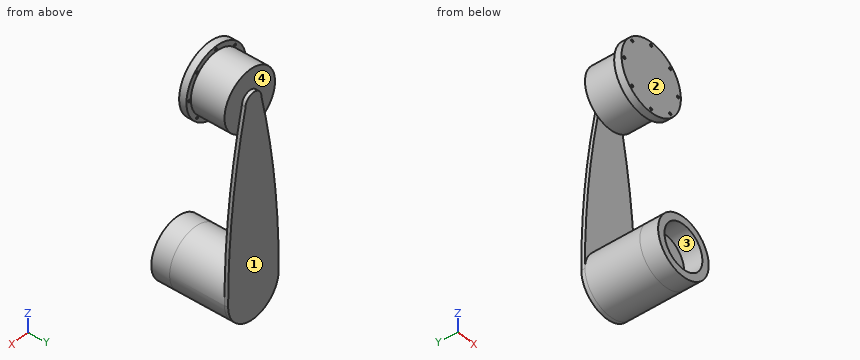
```python
from build123d import *
from build123d.topology import SkipClean

# Parameters (mm, degrees)
SKETCH_1_R          = 40
EXTRUDE_1_DEPTH     = 50
EXTRUDE_1_2_DEPTH   = 50
EXTRUDE_START       = 5
SKETCH_2_R          = 40
EXTRUDE_2_DEPTH     = 5
EXTRUDE_3_DEPTH     = 5
EXTRUDE_START_2     = -5
SKETCH_5_R          = 40
EXTRUDE_4_DEPTH     = 5
SKETCH_7_R          = 2
SKETCH_7_R_2        = 4
CUT_EXTRUDE_2_DEPTH = 10
CUT_EXTRUDE_START   = -59.05
SKETCH_9_R          = 40
CUT_EXTRUDE_4_DEPTH = 54.05
SKETCH_10_R         = 47
EXTRUDE_5_DEPTH     = 10
CUT_EXTRUDE_5_REACH = 302.04
SKETCH_11_R         = 1.75
CUT_EXTRUDE_START_2 = -80
SKETCH_12_R         = 39.999999969
CUT_EXTRUDE_6_DEPTH = 20
SKETCH_14_R         = 40
EXTRUDE_6_DEPTH     = 5
CUT_EXTRUDE_8_DEPTH = 10
CUT_EXTRUDE_9_DEPTH = 5
EXTRUDE_8_DEPTH     = 5
SKETCH_13_R         = 39.999999969
SKETCH_13_R_2       = 29.999999969
EXTRUDE_1_3_DEPTH   = 25


with BuildPart() as part:
    # Sketch 1 → Extrude 1 (new, symmetric)
    with BuildSketch(Plane(origin=(0, 0, 0), x_dir=(1, 0, 0), z_dir=(0, 1, 0))):
        with Locations(Location((0, 0, 0), (0, 0, 270))):
            Circle(SKETCH_1_R)
    extrude(amount=EXTRUDE_1_DEPTH, both=True)



with BuildPart() as body_2:
    # Sketch 1 → Extrude 1 2 (new, symmetric)
    with BuildSketch(Plane(origin=(0, 0, 0), x_dir=(1, 0, 0), z_dir=(0, 1, 0))):
        with Locations(Location((0, 250, 0), (0, 0, 270))):
            Circle(SKETCH_1_R)
    extrude(amount=EXTRUDE_1_2_DEPTH, both=True)


with BuildPart() as part_1:
    add(part.part)

    add(body_2.part)  # Extrude 2 merges body 2
    # Sketch 2 → Extrude 2 (add)
    with BuildSketch(Plane(origin=(0, 50, 0), x_dir=(1, 0, 0), z_dir=(0, 1, 0)).offset(EXTRUDE_START)):
        with BuildLine():
            ThreePointArc((39.999999755, 249.995569239), (-0.00221538, 210.000000061), (-40, 250))
            Line((-40, 250), (-40, 0))
            ThreePointArc((-40, 0), (-0.527343072, -39.996523715), (39.986095464, -1.054594484))
            Line((39.986095464, -1.054594484), (39.999999755, 249.995569239))
        make_face()
        with Locations(Location((0, 250, 0), (0, 0, 180))):
            Circle(SKETCH_2_R)
    extrude(amount=-EXTRUDE_2_DEPTH)

    # Sketch 3 → Extrude 3 (add)
    with BuildSketch(Plane(origin=(0, -50, 0), x_dir=(-1, 0, 0), z_dir=(0, -1, 0))):
        with BuildLine():
            Line((40, 0), (40, 250))
            ThreePointArc((40, 250), (0, 290), (-40, 250))
            Line((-40, 250), (-40, 0))
            ThreePointArc((-40, 0), (0, -40), (40, 0))
        make_face()
    extrude(amount=EXTRUDE_3_DEPTH)

    # Sketch 5 → Extrude 4 (add)
    with BuildSketch(Plane.XZ.offset(55).offset(EXTRUDE_START_2)):
        with Locations(Location((0, 0, 0), (0, 0, 180))):
            Circle(SKETCH_5_R)
    extrude(amount=EXTRUDE_4_DEPTH)

    # Sketch 7 → Cut-Extrude 2 (cut)
    with BuildSketch(Plane.XZ.offset(55)):
        with Locations(Location((17.25, -250, 0), (0, 0, 270))):
            Circle(SKETCH_7_R)
        with Locations(Location((8.625, -264.938938215, 0), (0, 0, 270))):
            Circle(SKETCH_7_R)
        with Locations(Location((-8.625, -264.938938215, 0), (0, 0, 270))):
            Circle(SKETCH_7_R)
        with Locations(Location((-17.25, -250, 0), (0, 0, 270))):
            Circle(SKETCH_7_R)
        with Locations(Location((-8.625, -235.061061785, 0), (0, 0, 270))):
            Circle(SKETCH_7_R)
        with Locations(Location((8.625, -235.061061785, 0), (0, 0, 270))):
            Circle(SKETCH_7_R)
        with Locations(Location((0, -250, 0), (0, 0, 270))):
            Circle(SKETCH_7_R_2)
    extrude(amount=-CUT_EXTRUDE_2_DEPTH, mode=Mode.SUBTRACT)

    # Sketch 9 → Cut-Extrude 4 (cut)
    with BuildSketch(Plane.XZ.offset(55).offset(CUT_EXTRUDE_START)):
        with Locations(Location((0, 0, 0), (0, 0, 270))):
            Circle(SKETCH_9_R)
    extrude(amount=CUT_EXTRUDE_4_DEPTH, mode=Mode.SUBTRACT)

    # Sketch 10 → Extrude 5 (add)
    with BuildSketch(Plane.XZ.offset(-4.05)):
        with Locations(Location((0, 0, 0), (0, 0, 270))):
            Circle(SKETCH_10_R)
    extrude(amount=EXTRUDE_5_DEPTH)

    # Sketch 11 → Cut-Extrude 5 (cut, up to next)
    with BuildSketch(Plane.XZ.offset(5.95), mode=Mode.PRIVATE) as cut_extrude_5_sk1:
        with Locations(Location((42.5, 0, 0), (0, 0, 270))):
            Circle(SKETCH_11_R)
    cut_extrude_5_tool1 = extrude(cut_extrude_5_sk1.sketch, amount=-CUT_EXTRUDE_5_REACH, mode=Mode.PRIVATE) & part_1.part
    # Sketch 11 → Cut-Extrude 5 (cut, up to next)
    with BuildSketch(Plane.XZ.offset(5.95), mode=Mode.PRIVATE) as cut_extrude_5_sk2:
        with Locations(Location((30.0520382, -30.0520382, 0), (0, 0, 270))):
            Circle(SKETCH_11_R)
    cut_extrude_5_tool2 = extrude(cut_extrude_5_sk2.sketch, amount=-CUT_EXTRUDE_5_REACH, mode=Mode.PRIVATE) & part_1.part
    # Sketch 11 → Cut-Extrude 5 (cut, up to next)
    with BuildSketch(Plane.XZ.offset(5.95), mode=Mode.PRIVATE) as cut_extrude_5_sk3:
        with Locations(Location((0, -42.5, 0), (0, 0, 270))):
            Circle(SKETCH_11_R)
    cut_extrude_5_tool3 = extrude(cut_extrude_5_sk3.sketch, amount=-CUT_EXTRUDE_5_REACH, mode=Mode.PRIVATE) & part_1.part
    # Sketch 11 → Cut-Extrude 5 (cut, up to next)
    with BuildSketch(Plane.XZ.offset(5.95), mode=Mode.PRIVATE) as cut_extrude_5_sk4:
        with Locations(Location((-30.0520382, -30.0520382, 0), (0, 0, 270))):
            Circle(SKETCH_11_R)
    cut_extrude_5_tool4 = extrude(cut_extrude_5_sk4.sketch, amount=-CUT_EXTRUDE_5_REACH, mode=Mode.PRIVATE) & part_1.part
    # Sketch 11 → Cut-Extrude 5 (cut, up to next)
    with BuildSketch(Plane.XZ.offset(5.95), mode=Mode.PRIVATE) as cut_extrude_5_sk5:
        with Locations(Location((-42.5, 0, 0), (0, 0, 270))):
            Circle(SKETCH_11_R)
    cut_extrude_5_tool5 = extrude(cut_extrude_5_sk5.sketch, amount=-CUT_EXTRUDE_5_REACH, mode=Mode.PRIVATE) & part_1.part
    # Sketch 11 → Cut-Extrude 5 (cut, up to next)
    with BuildSketch(Plane.XZ.offset(5.95), mode=Mode.PRIVATE) as cut_extrude_5_sk6:
        with Locations(Location((-30.0520382, 30.0520382, 0), (0, 0, 270))):
            Circle(SKETCH_11_R)
    cut_extrude_5_tool6 = extrude(cut_extrude_5_sk6.sketch, amount=-CUT_EXTRUDE_5_REACH, mode=Mode.PRIVATE) & part_1.part
    # Sketch 11 → Cut-Extrude 5 (cut, up to next)
    with BuildSketch(Plane.XZ.offset(5.95), mode=Mode.PRIVATE) as cut_extrude_5_sk7:
        with Locations(Location((0, 42.5, 0), (0, 0, 270))):
            Circle(SKETCH_11_R)
    cut_extrude_5_tool7 = extrude(cut_extrude_5_sk7.sketch, amount=-CUT_EXTRUDE_5_REACH, mode=Mode.PRIVATE) & part_1.part
    # Sketch 11 → Cut-Extrude 5 (cut, up to next)
    with BuildSketch(Plane.XZ.offset(5.95), mode=Mode.PRIVATE) as cut_extrude_5_sk8:
        with Locations(Location((30.0520382, 30.0520382, 0), (0, 0, 270))):
            Circle(SKETCH_11_R)
    cut_extrude_5_tool8 = extrude(cut_extrude_5_sk8.sketch, amount=-CUT_EXTRUDE_5_REACH, mode=Mode.PRIVATE) & part_1.part
    add(cut_extrude_5_tool1.solids().sort_by_distance((42.5, -5.95, 0))[0], mode=Mode.SUBTRACT)
    add(cut_extrude_5_tool2.solids().sort_by_distance((30.052038, -5.95, -30.052038))[0], mode=Mode.SUBTRACT)
    add(cut_extrude_5_tool3.solids().sort_by_distance((0, -5.95, -42.5))[0], mode=Mode.SUBTRACT)
    add(cut_extrude_5_tool4.solids().sort_by_distance((-30.052038, -5.95, -30.052038))[0], mode=Mode.SUBTRACT)
    add(cut_extrude_5_tool5.solids().sort_by_distance((-42.5, -5.95, 0))[0], mode=Mode.SUBTRACT)
    add(cut_extrude_5_tool6.solids().sort_by_distance((-30.052038, -5.95, 30.052038))[0], mode=Mode.SUBTRACT)
    add(cut_extrude_5_tool7.solids().sort_by_distance((0, -5.95, 42.5))[0], mode=Mode.SUBTRACT)
    add(cut_extrude_5_tool8.solids().sort_by_distance((30.052038, -5.95, 30.052038))[0], mode=Mode.SUBTRACT)

    # Sketch 12 → Cut-Extrude 6 (cut)
    with BuildSketch(Plane(origin=(0, 55, 0), x_dir=(1, 0, 0), z_dir=(0, 1, 0)).offset(CUT_EXTRUDE_START_2)):
        with Locations(Location((0, 250, 0), (0, 0, 180))):
            Circle(SKETCH_12_R)
    extrude(amount=-CUT_EXTRUDE_6_DEPTH, mode=Mode.SUBTRACT)


with BuildPart() as cut_extrude_6_piece_1:
    # of the separate pieces the step leaves, piece 1, a body of its own (cut_extrude_6_pieces)
    add(part_1.part.solids().sort_by_distance((0, 4.05, -47))[0])

    # Sketch 14 → Extrude 6 (add)
    with BuildSketch(Plane.XZ.offset(-50)):
        with Locations(Location((0, -250, 0), (0, 0, 180))):
            Circle(SKETCH_14_R)
    extrude(amount=-EXTRUDE_6_DEPTH)

    # Sketch 17 → Cut-Extrude 9 (cut)
    with BuildSketch(Plane(origin=(0, 55, 0), x_dir=(1, 0, 0), z_dir=(0, 1, 0))):
        with BuildLine():
            Line((-40, 0), (-40, 250))
            ThreePointArc((-40, 250), (0, 290), (40, 250))
            Line((40, 250), (40, 0))
            ThreePointArc((40, 0), (0, -40), (-40, 0))
        make_face()
    extrude(amount=-CUT_EXTRUDE_9_DEPTH, mode=Mode.SUBTRACT)


with BuildPart() as cut_extrude_6_piece_2:
    # of the separate pieces the step leaves, piece 2, a body of its own (cut_extrude_6_pieces)
    add(part_1.part.solids().sort_by_distance((0, -45, -210.000000015))[0])

    # Sketch 15 → Cut-Extrude 8 (cut)
    with BuildSketch(Plane.XZ.offset(55)):
        with BuildLine():
            Line((40, 0), (40, -250))
            ThreePointArc((40, -250), (0, -290), (-40, -250))
            Line((-40, -250), (-40, 0))
            ThreePointArc((-40, 0), (0, 40), (40, 0))
        make_face()
    extrude(amount=-CUT_EXTRUDE_8_DEPTH, mode=Mode.SUBTRACT)


with BuildPart() as cut_extrude_9_piece_1:
    # of the separate pieces the step leaves, piece 1, a body of its own (cut_extrude_9_pieces)
    add(cut_extrude_6_piece_1.part.solids().sort_by_distance((0, 50, -210))[0])



with BuildPart() as cut_extrude_9_piece_2:
    # of the separate pieces the step leaves, piece 2, a body of its own (cut_extrude_9_pieces)
    add(cut_extrude_6_piece_1.part.solids().sort_by_distance((0, 4.05, -47))[0])


with BuildPart() as cut_extrude_9_piece_1_1:
    add(cut_extrude_9_piece_1.part)

    add(cut_extrude_9_piece_2.part)  # Extrude 8 merges Cut-Extrude 9 piece 2
    # Sketch 18 → Extrude 8 (add)
    with BuildSketch(Plane(origin=(0, 55, 0), x_dir=(1, 0, 0), z_dir=(0, 1, 0))):
        with BuildLine():
            ThreePointArc((40.000000061, 250), (0, 290.000000061), (-40.000000061, 250))
            ThreePointArc((-40.000000061, 250), (-33.286999063, 124.225930105), (-12.5, 0))
            ThreePointArc((-12.5, 0), (0, -12.5), (12.5, 0))
            ThreePointArc((12.5, 0), (33.286999063, 124.225930105), (40.000000061, 250))
        make_face()
    extrude(amount=-EXTRUDE_8_DEPTH)

    # Sketch 13 → Extrude 1 3 (add)
    with SkipClean():  # the faces are left unmerged after this step: merging them gives an invalid solid
        with BuildSketch(Plane.XZ.offset(25)):
            with Locations((0, -250)):
                Circle(SKETCH_13_R)
            with Locations((0, -250)):
                Circle(SKETCH_13_R_2, mode=Mode.SUBTRACT)
        extrude(amount=EXTRUDE_1_3_DEPTH)
    add(cut_extrude_9_piece_1_1.part.scale(1), mode=Mode.REPLACE)  # the faces are merged on a copy


solid = cut_extrude_9_piece_1_1.part
```
Build history of the part. All positions in model axes, mm. Face numbers are marked on the shaded views. A direction names the side the tool comes from. Round coordinates to 2 decimals unless told otherwise and drop trailing zeros. Order: outer loops, then holes, each group sorted by start corner. A loop starts at its lowest first (then second) coordinate and runs counter-clockwise, first axis right, second up. Notation, with made-up numbers: (-23, 64.5) -> (18, 64.5) arc R15 ccw to (18, 75.5) -> close; hole circle Ø1 at (67.25, 16.5). An arc over 180 degrees is marked (long way). Answer in a Markdown table with one row per item.
1) Band-saw the part on A-A on y = -1.5. Give the number of separate pieces and of enclosed holes in the cut face, and give its area (3 significant figures).
Values:
| item | result |
|---|---|
| separate pieces | 2 |
| enclosed holes | 8 |
| area | 11,900 mm2 |
2) Band-saw the part on C-C on x = -7. Give the cut face in (y, z), and give its area (3 significant figures).
Values:
| item | result |
|---|---|
| outline | (-50, -289.38) -> (55, -289.38) -> (55, 10.36) -> (50, 10.36) -> (50, 39.38) -> (4.05, 39.38) -> (4.05, 46.48) -> (-5.95, 46.48) -> (-5.95, -46.48) -> (4.05, -46.48) -> (4.05, -39.38) -> (50, -39.38) -> (50, -210.62) -> (-50, -210.62) -> (-50, -220.83) -> (-25, -220.83) -> (-25, -279.17) -> (-50, -279.17) -> close |
| area | 12,500 mm2 |
3) Wall check: L1, parallel to X at y = -0.5, z = 0; L2, parallel to Z at x = -1, y = 12.5; L3, parallel to Y at x = -4.5, z = -45.5. Give the ranges that are in metal, low to high.
Values:
| item | result |
|---|---|
| L1 | -47 to -44.25, -40.75 to 40.75, 44.25 to 47 |
| L2 | -289.99 to -210.01, -39.99 to 39.99 |
| L3 | -5.95 to 4.05, 50 to 55 |
4) Which spindle directions (+Z, -Z, +X, -X, +Y, -Y) get a long thin tool onto all of the face, cutting with end or side? Do the marked faces 1 and 2. Say none if no direction does.
Values:
| item | result |
|---|---|
| face 1 | +Z, -Z, +X, -X, +Y |
| face 2 | +Z, +X, -X, -Y |
5) Mould opens along Z. For the marked faces 3 and 4 say: released by +Z, released by -Z, zero draft, split by the parting line, or undercut.
Values:
| item | result |
|---|---|
| face 3 | undercut |
| face 4 | zero draft |
6) Band-saw the part on B-B on y = 39. Give the cut face in (x, z), and give its area (3 significant figures).
Values:
| item | result |
|---|---|
| outline | circle Ø80 at (0, -250); circle Ø80 at (0, 0) |
| area | 10,100 mm2 |
7) Pin check, flat tips, straight feed: P1, Ø4, axis at y = 14, z = -26.5, coming from the +X side; P2, Ø4.5, axis at x = -42.5, z = 0, coming from the +Y side; P3, Ø1.5, axis at x = -8.5, y = -20, coming from the +Z side. Stop position of each tip, or through.
Values:
| item | result |
|---|---|
| P1 | x = 31.62 |
| P2 | y = 4.05 |
| P3 | z = -210.76 |
8) Band-saw the part on D-D on z = -233.5. Give the cut face in (x, y).
Values:
| item | result |
|---|---|
| outline | (-39.93, 50) -> (-36.44, 50) -> (-36.44, -50) -> (-25.05, -50) -> (-25.05, -25) -> (25.05, -25) -> (25.05, -50) -> (36.44, -50) -> (36.44, 50) -> (39.93, 50) -> (39.93, 55) -> (-39.93, 55) -> close |
